from build123d import *

# Parameters (mm, degrees)
SKETCH_1_W               = 57
SKETCH_1_H               = 57
EXTRUDE_1_DEPTH          = 5
SKETCH_2_R               = 23.5
CUT_EXTRUDE_1_DEPTH      = 2
SKETCH_3_R               = 25.1
CUT_EXTRUDE_2_DEPTH      = 3
SKETCH_4_R               = 2.5
SKETCH_4_R_2             = 1.7
CUT_EXTRUDE_3_DEPTH      = 41.614036982
CUT_EXTRUDE_4_DEPTH      = 3
CUT_EXTRUDE_5_DEPTH      = 1.1
PATTERN_CIRCULAR_1_COUNT = 4
FILLET_1_R               = 5


with BuildPart() as part:
    # 草图1 → 凸台-拉伸1 (new body)
    with BuildSketch(Plane(origin=(0, 0, 0), x_dir=(1, 0, 0), z_dir=(0, 1, 0))):
        Rectangle(SKETCH_1_W, SKETCH_1_H)
    extrude(amount=EXTRUDE_1_DEPTH)

    # 草图2 → 切除-拉伸1 (cut)
    with BuildSketch(Plane(origin=(0, 5, 0), x_dir=(1, 0, 0), z_dir=(0, 1, 0))):
        with Locations(Location((0, 0, 0), (0, 0, 270))):
            Circle(SKETCH_2_R)
    extrude(amount=-CUT_EXTRUDE_1_DEPTH, mode=Mode.SUBTRACT)

    # 草图3 → 切除-拉伸2 (cut)
    with BuildSketch(Plane(origin=(0, 3, 0), x_dir=(1, 0, 0), z_dir=(0, 1, 0))):
        with Locations(Location((0, 0, 0), (0, 0, 270))):
            Circle(SKETCH_3_R)
    extrude(amount=-CUT_EXTRUDE_2_DEPTH, mode=Mode.SUBTRACT)

    # 草图4 → 切除-拉伸3 (cut, through all)
    with BuildSketch(Plane(origin=(0, 5, 0), x_dir=(1, 0, 0), z_dir=(0, 1, 0))):
        with Locations(Location((-23.5, 23.5, 0), (0, 0, 270))):
            Circle(SKETCH_4_R)
        with Locations(Location((-15.5, 25, 0), (0, 0, 270))):
            Circle(SKETCH_4_R_2)
    cut_extrude_3 = extrude(amount=-CUT_EXTRUDE_3_DEPTH, mode=Mode.SUBTRACT)

    # 草图5 → 切除-拉伸4 (cut)
    with BuildSketch(Plane(origin=(0, 5, 0), x_dir=(1, 0, 0), z_dir=(0, 1, 0))):
        with BuildLine():
            Line((-18.5, 25), (-18.5, 30.780907879))
            ThreePointArc((-18.5, 30.780907879), (-15.5, 33.780907879), (-12.5, 30.780907879))
            Line((-12.5, 30.780907879), (-12.5, 25))
            ThreePointArc((-12.5, 25), (-15.5, 22), (-18.5, 25))
        make_face()
    cut_extrude_4 = extrude(amount=-CUT_EXTRUDE_4_DEPTH, mode=Mode.SUBTRACT)

    # 草图6 → 切除-拉伸5 (cut)
    with BuildSketch(Plane.XZ):
        Polygon((-28.5, 11.1), (-28.5, -11.1), (-27.5, -10.1), (-27.5, 10.1), align=None)
    cut_extrude_5 = extrude(amount=-CUT_EXTRUDE_5_DEPTH, mode=Mode.SUBTRACT)

    # 阵列(圆周)1: 切除-拉伸3, 切除-拉伸4, 切除-拉伸5 ×4 about axis
    pattern_circular_1_axis = Axis((0, 0, 0), (0, 1, 0))
    add([cut_extrude_3.rotate(pattern_circular_1_axis, i * 360 / PATTERN_CIRCULAR_1_COUNT) for i in range(1, PATTERN_CIRCULAR_1_COUNT)], mode=Mode.SUBTRACT)
    add([cut_extrude_4.rotate(pattern_circular_1_axis, i * 360 / PATTERN_CIRCULAR_1_COUNT) for i in range(1, PATTERN_CIRCULAR_1_COUNT)], mode=Mode.SUBTRACT)
    add([cut_extrude_5.rotate(pattern_circular_1_axis, i * 360 / PATTERN_CIRCULAR_1_COUNT) for i in range(1, PATTERN_CIRCULAR_1_COUNT)], mode=Mode.SUBTRACT)

    # 圆角1
    fillet_1_edges = [part.edges().sort_by_distance(p)[0] for p in [
        (28.5, 2.5, 28.5),
        (-28.5, 2.5, 28.5),
        (-28.5, 2.5, -28.5),
        (28.5, 2.5, -28.5),
    ]]
    fillet(fillet_1_edges, radius=FILLET_1_R)


solid = part.part
CAD build for the part. Positions are in the model's coordinates, mm. A direction names the side the tool comes from. Round coordinates to 2 decimals unless told otherwise and drop trailing zeros. Loops run counter-clockwise (first coordinate to the right, second up) from the corner with the lowest first, then second, coordinate; pieces in that order, holes last. Notation, with made-up numbers: M -38,-19.75 L -4,-19.75 A31 cw -4,8.25 Z; hole C 7.5,-19.5 d6. An arc over 180 degrees is marked long. One line per question, with ' | ' between items. Start each with the question number.
Item 1: Cut at A-A, the plane z = 0. Write the cut outline in (x, y).
Item 2: Cut at C-C, the plane x = -1. Write the cut outline in (y, z), plus the area to 3 significant figures.
Item 3: Wall check: line 1 (Z direction, x = -0.5, y = 2.05); line 2 (X direction, y = 4.55, z = 3); line 3 (Z direction, x = -7, y = 4.2). Give the ranges that are in metal, low to high.
Item 4: Two-plate mould, pull along Z, no slides. Class faces 1 (the cylindrical face through (-22, 3.5, 15.4)), 2 (the flat face through (-12.5, 4, -27)), 3 (the cylindrical face through (15.4, 3.5, 22)): pulls with the +Z half, pulls with the -Z half, needs draft (parallel to the pull), parting line crosses it, or undercut.
Item 5: Pin check, flat tips, straight feed: pin 1 Ø2.5 at (x, y) = (26, 3) entering from +Z; pin 2 Ø4.5 at (x, z) = (25, -15.5) entering from +Y; pin 3 Ø2.5 at (y, z) = (4, -26.5) entering from +X. Stop position of each tip, or through.
Item 6: Cut at D-D, the plane z = -15.5. Write the cut outline in (x, y).
Item 7: Cut at B-B, the plane y = 4.1. State how many separate pieces and enclosed holes the cut face has, plus the area to 3 significant figures.
Item 8: Which spindle directions (+Z, -Z, +X, -X, +Y, -Y) get a long thin tool onto all of the face, cutting with end or side? Do faces 4 (the flat face through (12.5, 4, 27)), 5 (the flat face through (-27, 2, 15)), 6 (the flat face through (-15, 2, -27)). Say none if no direction does.
Responses:
1) outline: M -28.5,1.1 L -27.5,1.1 L -27.5,0 L -25.1,0 L -25.1,3 L -23.5,3 L -23.5,5 L -28.5,5 Z; M 23.5,3 L 25.1,3 L 25.1,0 L 27.5,0 L 27.5,1.1 L 28.5,1.1 L 28.5,5 L 23.5,5 Z
2) outline: M 0,-27.5 L 1.1,-27.5 L 1.1,-28.5 L 5,-28.5 L 5,-23.48 L 3,-23.48 L 3,-25.08 L 0,-25.08 Z; M 0,25.08 L 3,25.08 L 3,23.48 L 5,23.48 L 5,28.5 L 1.1,28.5 L 1.1,27.5 L 0,27.5 Z | area: 38.4 mm²
3) line 1: z = -28.5 to -25.1, 25.1 to 28.5 | line 2: x = -28.5 to -23.31, 23.31 to 28.5 | line 3: z = -28.5 to -22.43, 22.43 to 28.5
4) face 1: undercut | face 2: needs draft | face 3: pulls with the +Z half
5) pin 1: stops at z = 28.34 | pin 2: stops at y = 2 | pin 3: stops at x = 28.18
6) outline: M -28.5,0 L -19.74,0 L -19.74,3 L -17.66,3 L -17.66,5 L -28.5,5 Z; M 17.66,3 L 19.74,3 L 19.74,0 L 23.3,0 L 23.3,2 L 22,2 L 22,5 L 17.66,5 Z; M 26.7,0 L 28.5,0 L 28.5,2 L 26.7,2 Z
7) separate pieces: 1 | enclosed holes: 5 | area: 1,270 mm²
8) face 4: +Z, +Y | face 5: -X, +Y | face 6: -Z, +Y
